CAD build for the part. Positions are in the model's coordinates, mm. A direction names the side the tool comes from. Coordinates: 2 decimals unless noted, no trailing zeros. Order: outer loops, then holes, each group sorted by start corner. A loop starts at its lowest first (then second) coordinate and runs counter-clockwise, first axis right, second up. Notation, with made-up numbers: M -35.5,33 L 13.5,33 A21 cw 13.5,58 Z; hole C 24,-2 d7. An arc over 180 degrees is marked long. Write item = value, one per line.
from build123d import *

# Parameters (mm, degrees)
SKETCH_1_W           = 145
SKETCH_1_H           = 120
SKETCH_1_R           = 1.6
EXTRUDE_1_DEPTH      = 5
SKETCH_2_W           = 145
SKETCH_2_H           = 5
CUT_EXTRUDE_1_DEPTH  = 8
SKETCH_3_W           = 145
SKETCH_3_H           = 115
SKETCH_3_W_2         = 135
SKETCH_3_H_2         = 107
EXTRUDE_6_DEPTH      = 30
SKETCH_4_W           = 145
SKETCH_4_H           = 3
EXTRUDE_7_DEPTH      = 41.25
SKETCH_7_W           = 9
SKETCH_7_H           = 18
CUT_EXTRUDE_4_DEPTH  = 7
SKETCH_8_W           = 30
SKETCH_8_H           = 6
CUT_EXTRUDE_6_DEPTH  = 6
SKETCH_9_W           = 6.5
SKETCH_9_H           = 9
CUT_EXTRUDE_7_DEPTH  = 6
SKETCH_6_W           = 17.5
SKETCH_6_H           = 17
CUT_EXTRUDE_8_DEPTH  = 10
SKETCH_11_R          = 1.7
SKETCH_11_W          = 108
SKETCH_11_H          = 68.7
CUT_EXTRUDE_9_DEPTH  = 5
FILLET_1_R           = 5
FILLET_2_R           = 5
SKETCH_13_R          = 1.65
CUT_EXTRUDE_10_DEPTH = 8


with BuildPart() as part:
    # 草图1 → 凸台-拉伸1 (new body)
    with BuildSketch(Plane.XY):
        Rectangle(SKETCH_1_W, SKETCH_1_H)
        with Locations((-49.95, -23.5)):
            Circle(SKETCH_1_R, mode=Mode.SUBTRACT)
        with Locations((-49.95, 31.5)):
            Circle(SKETCH_1_R, mode=Mode.SUBTRACT)
        with Locations((-61.35, 46.25)):
            Circle(SKETCH_1_R, mode=Mode.SUBTRACT)
        with Locations((61.35, -46.6)):
            Circle(SKETCH_1_R, mode=Mode.SUBTRACT)
        with Locations((61.35, 46.6)):
            Circle(SKETCH_1_R, mode=Mode.SUBTRACT)
        with Locations((-61.35, -46.25)):
            Circle(SKETCH_1_R, mode=Mode.SUBTRACT)
        with Locations((62.35, 31.5)):
            Circle(SKETCH_1_R, mode=Mode.SUBTRACT)
        with Locations((62.35, -23.5)):
            Circle(SKETCH_1_R, mode=Mode.SUBTRACT)
    extrude(amount=EXTRUDE_1_DEPTH)

    # 草图2 → 切除-拉伸1 (cut)
    with BuildSketch(Plane.XY.offset(5)):
        with Locations((0, -57.5)):
            Rectangle(SKETCH_2_W, SKETCH_2_H)
    extrude(amount=-CUT_EXTRUDE_1_DEPTH, mode=Mode.SUBTRACT)

    # 草图3 → 凸台-拉伸6 (add)
    with BuildSketch(Plane.XY.offset(5)):
        with Locations((0, 2.5)):
            Rectangle(SKETCH_3_W, SKETCH_3_H)
        with Locations((0, 1.5)):
            Rectangle(SKETCH_3_W_2, SKETCH_3_H_2, mode=Mode.SUBTRACT)
    extrude(amount=-EXTRUDE_6_DEPTH)

    # 草图4 → 凸台-拉伸7 (add)
    with BuildSketch(Plane(origin=(0, -55, 0), x_dir=(-1, 0, 0), z_dir=(0, -1, 0))):
        with Locations((0, 23.5)):
            Rectangle(SKETCH_4_W, SKETCH_4_H)
    extrude(amount=EXTRUDE_7_DEPTH)

    # 草图7 → 切除-拉伸4 (cut)
    with BuildSketch(Plane(origin=(72.5, 0, 0), x_dir=(0, 0, -1), z_dir=(1, 0, 0))):
        with Locations((15.8, 21)):
            Rectangle(SKETCH_7_W, SKETCH_7_H)
    extrude(amount=-CUT_EXTRUDE_4_DEPTH, mode=Mode.SUBTRACT)

    # 草图8 → 切除-拉伸6 (cut)
    with BuildSketch(Plane.XZ.offset(55)):
        with Locations((27.5, -16)):
            Rectangle(SKETCH_8_W, SKETCH_8_H)
    extrude(amount=-CUT_EXTRUDE_6_DEPTH, mode=Mode.SUBTRACT)

    # 草图9 → 切除-拉伸7 (cut)
    with BuildSketch(Plane(origin=(72.5, 0, 0), x_dir=(0, 0, -1), z_dir=(1, 0, 0))):
        with Locations((15.75, -37.5)):
            Rectangle(SKETCH_9_W, SKETCH_9_H)
    extrude(amount=-CUT_EXTRUDE_7_DEPTH, mode=Mode.SUBTRACT)

    # 草图6 → 切除-拉伸8 (cut)
    with BuildSketch(Plane.XZ.offset(55)):
        with Locations((-37.94, -11.5)):
            Rectangle(SKETCH_6_W, SKETCH_6_H)
    extrude(amount=-CUT_EXTRUDE_8_DEPTH, mode=Mode.SUBTRACT)

    # 草图11 → 切除-拉伸9 (cut)
    with BuildSketch(Plane.XY.offset(5)):
        with Locations((56.8, 33.8)):
            Circle(SKETCH_11_R)
        with Locations(Location((56.8, -33.8, 0), (0, 0, 180))):
            Circle(SKETCH_11_R)
        with Locations((-56.8, -33.8)):
            Circle(SKETCH_11_R)
        with Locations(Location((-56.8, 33.8, 0), (0, 0, 180))):
            Circle(SKETCH_11_R)
        Rectangle(SKETCH_11_W, SKETCH_11_H)
    extrude(amount=-CUT_EXTRUDE_9_DEPTH, mode=Mode.SUBTRACT)

    # 圆角1
    fillet_1_edges = [part.edges().sort_by_distance(p)[0] for p in [
        (0, -55, 5),
    ]]
    fillet(fillet_1_edges, radius=FILLET_1_R)

    # 圆角2
    fillet_2_edges = [part.edges().sort_by_distance(p)[0] for p in [
        (0, 60, 5),
    ]]
    fillet(fillet_2_edges, radius=FILLET_2_R)

    # 草图13 → 切除-拉伸10 (cut)
    with BuildSketch(Plane.XY.offset(-22)):
        with Locations((-62.5, -86.25)):
            Circle(SKETCH_13_R)
        with Locations((62.5, -86.25)):
            Circle(SKETCH_13_R)
    extrude(amount=-CUT_EXTRUDE_10_DEPTH, mode=Mode.SUBTRACT)


solid = part.part
(1) Slice it at B-B, the plane x = -20.5. Write the cut outline in (y, z).
Evaluation:
outline = M -96.25,-25 L -52,-25 L -52,0 L -34.35,0 L -34.35,5 L -50,5 A5 ccw -55,0 L -55,-22 L -96.25,-22 Z; M 34.35,0 L 55,0 L 55,-25 L 60,-25 L 60,0 A5 ccw 55,5 L 34.35,5 Z
(2) Slice it at D-D, the plane x = -41. Write the cut outline in (y, z).
Evaluation:
outline = M -96.25,-25 L -52,-25 L -52,-20 L -55,-20 L -55,-22 L -96.25,-22 Z; M -55,-3 L -52,-3 L -52,0 L -34.35,0 L -34.35,5 L -50,5 A5 ccw -55,0 Z; M 34.35,0 L 55,0 L 55,-25 L 60,-25 L 60,0 A5 ccw 55,5 L 34.35,5 Z
(3) Wall check: line 1 (X direction, y = -86.25, z = -23); line 2 (Y direction, x = 62.5, z = -23); line 3 (X direction, y = -22, z = -9.5). Give the ranges that are in metal, low to high. Write a range as from..to.
Evaluation:
line_1 = -72.5..-64.15, -60.85..60.85, 64.15..72.5
line_2 = -96.25..-87.9, -84.6..-52, 55..60
line_3 = -72.5..-67.5, 67.5..72.5
(4) Slice it at A-A, the plane y = -38.5. Write the cut outline in (x, z), then the cut area to 4 significant figures.
Evaluation:
outline = M -72.5,-25 L -67.5,-25 L -67.5,0 L 67.5,0 L 67.5,-12.5 L 72.5,-12.5 L 72.5,5 L -72.5,5 Z; M 67.5,-25 L 72.5,-25 L 72.5,-19 L 67.5,-19 Z
area = 942.5 mm²
(5) Pin check, flat tips, straight feed: pin 1 Ø1 at (x, y) = (25, -59) entering from +Z; pin 2 Ø1.5 at (x, y) = (30.5, -53.5) entering from +Z; pin 3 Ø1.5 at (x, z) = (21, 3.5) entering from -Y; pin 4 Ø1.9 at (x, y) = (61.35, -46.6) entering from +Z. Stop position of each tip, or through.
Evaluation:
pin_1 = -22
pin_2 = 4.18
pin_3 = -54.18
pin_4 = through
(6) Slice it at C-C, the plane y = 21. Write the cut outline in (x, z), then the cut area to 3 significant figures.
Evaluation:
outline = M -72.5,-25 L -67.5,-25 L -67.5,0 L -54,0 L -54,5 L -72.5,5 Z; M 54,0 L 67.5,0 L 67.5,-11.3 L 72.5,-11.3 L 72.5,5 L 54,5 Z; M 67.5,-25 L 72.5,-25 L 72.5,-20.3 L 67.5,-20.3 Z
area = 390 mm²
(7) Tool access for faces 1 (the face through (-1, 34.35, 3)), 2 (the face through (-67.5, 1, -12)), 3 (the face through (1, -54, 3)), 4 (the face through (-1, 60, -13)), 5 (the face through (70, -33, -16)): list every direction of +Z, -Z, +X, -X, +Y, -Y with a clear straight run to the whole face (end or side of a thin tool).
Evaluation:
face_1 = +Z, -Z
face_2 = -Z
face_3 = +Z, +X, -X, -Y
face_4 = +Z, -Z, +X, -X, +Y
face_5 = +X
(8) Pull direction Z, two halves, no side cores. Call faces 6 (the face through (1, -75, -22)), 7 (the face through (70, 12, -16)), 8 (the face through (67.5, 1, -12)): +Z half, -Z half, draft (parallel to the pull), parting line (faces both ways), or undercut.
Evaluation:
face_6 = +Z half
face_7 = undercut
face_8 = draft
